Model file for the job. Use its own axes, mm. Give positions to 0.01 mm unless a question says otherwise; leave off trailing zeros. Write each loop counter-clockwise with the first axis right and the second up, starting at its lowest first coordinate (ties: lowest second). Pieces come first, ordered by that corner, then holes.
```python
from build123d import *

# Parameters (mm, degrees)
CYLINDER020_W               = 6
CYLINDER020_H               = 10
CYLINDER020_ANGLE           = 120
CYLINDER020_PLACEMENT_ANGLE = 30
CYLINDER015_W               = 8
CYLINDER015_H               = 10
CYLINDER015_ANGLE           = 120
CYLINDER015_PLACEMENT_ANGLE = 30


with BuildPart() as cilindro011:
    # Cylinder020 → Cylinder020 (revolve)
    with BuildSketch(Plane.XZ):
        with Locations((3, 5)):
            Rectangle(CYLINDER020_W, CYLINDER020_H)
    revolve(axis=Axis((0, 0, 0), (0, 0, 1)), revolution_arc=CYLINDER020_ANGLE)


with BuildPart() as cilindro011_1:
    # Cylinder020 placement: moved
    add(cilindro011.part.moved(Location((-30.75, -30, 0))).rotate(Axis((-30.75, -30, 0), (0, 0, 1)), CYLINDER020_PLACEMENT_ANGLE))


with BuildPart() as obj1:
    # Cylinder015 → Cylinder015 (revolve)
    with BuildSketch(Plane.XZ):
        with Locations((4, 5)):
            Rectangle(CYLINDER015_W, CYLINDER015_H)
    revolve(axis=Axis((0, 0, 0), (0, 0, 1)), revolution_arc=CYLINDER015_ANGLE)


with BuildPart() as obj1_1:
    # Cylinder015 placement: moved
    add(obj1.part.moved(Location((-30.75, -30, 0))).rotate(Axis((-30.75, -30, 0), (0, 0, 1)), CYLINDER015_PLACEMENT_ANGLE))

    # Cut005: cut Cilindro011
    add(cilindro011_1.part, mode=Mode.SUBTRACT)


solid = obj1_1.part
```
1. Slice it at A-A, the plane y = -26.15. Write the cut outline in (x, z), and give its area (3 significant figures).
Calculated:
outline: (-37.42, 0) - (-35.35, 0) - (-35.35, 10) - (-37.42, 10) - close; (-26.15, 0) - (-24.08, 0) - (-24.08, 10) - (-26.15, 10) - close
area: 41.3 mm2
2. Pin check, flat tips, straight feed: P1, Ø3, axis at y = -26, z = 7, coming from the -X side; P2, Ø1.5, axis at x = -29.5, z = 6.5, coming from the -Y side. Stop position of each tip, or through.
Calculated:
P1: stops at x = -37.68
P2: stops at y = -24.34
3. Pull direction X, two halves, no side cores. Call faces 1 (the cylindrical face through (-30.7, -24, 5.1)), 2 (the flat face through (-24.7, -26.507, 5.07)), 3 (the flat face through (-36.8, -26.507, 5.07)): +X half, -X half, draft (parallel to the pull), parting line (faces both ways), or undercut.
Calculated:
face 1: undercut
face 2: +X half
face 3: -X half
4. Slice it at D-D, the plane y = -24.4. Write the cut outline in (x, z).
Calculated:
outline: (-36.46, 0) - (-32.9, 0) - (-32.9, 10) - (-36.46, 10) - close; (-28.6, 0) - (-25.04, 0) - (-25.04, 10) - (-28.6, 10) - close
5. Slice it at B-B, the plane z = 7.75. Write the cut outline in (x, y).
Calculated:
outline: (-37.68, -26) - (-35.95, -27) arc R6 cw to (-25.55, -27) - (-23.82, -26) arc R8 ccw to start
6. Probe probe 1 along X at (y, z) = (-25.3, 1.5); probe 2 along X at (y, z) = (-25.85, 4.5); probe 3 along Y at (x, z) = (-36, 1.25). List the from-to ranges inside material, lowest first.
Calculated:
probe 1: x = -37.22 to -34.48, -27.02 to -24.28
probe 2: x = -37.59 to -35.08, -26.42 to -23.91
probe 3: y = -26.97 to -23.96
7. Slice it at C-C, the plane y = -23.6. Write the cut outline in (x, z), and give its area (3 significant figures).
Calculated:
outline: (-35.55, 0) - (-25.95, 0) - (-25.95, 10) - (-35.55, 10) - close
area: 96.0 mm2
